Design review of the part shown in the three views and the two pictorial views. Dimensions are in mm from the part's minimum x, y and z. A direction names the side the tool comes from. Round coordinates to 2 decimals unless told otherwise and drop trailing zeros. Loops run counter-clockwise (first coordinate to the right, second up) from the corner with the lowest first, then second, coordinate; pieces in that order, holes last.
1. Consider section C-C on x = 8.25. State the section outline as (y, z) points.
2. Consider section B-B on x = 18. State the section outline as (y, z) points.
3. Clearance check with flat-ended pins moving along their axes: pin 1 Ø2.5 at (y, z) = (13, 5) entering from -X; pin 2 Ø2.5 at (x, z) = (19, 3) entering from +Y. State where each tip first meets the part, or that it passes through.
4. Consider section A-A on z = 5. State the section outline as (x, y) points, then the cut area to 3 significant figures.
5. Draft analysis for pull direction Z (two halves, no side actions). For the marked faces 4, 5 and 6, state which applies: released by +Z, released by -Z, zero draft, split by the parting line, or undercut.
6. Tool access review of the marked faces 1, 2 and 3: name each direction out of +Z, -Z, +X, -X, +Y, -Y from which nothing blocks a thin tool from reaching the whole face with its end or side.
7. To check wall thickness, follow line 1 along X through (y, z) = (3.8, 5); line 2 along Z through (x, y) = (18, 3.4); line 3 along Y through (x, z) = (11.5, 5). State the ranges of each line that lie inside material, in increasing order.
8. Consider section D-D on y = 13. State the section outline as (x, z) points, then the cut area to 3 significant figures.
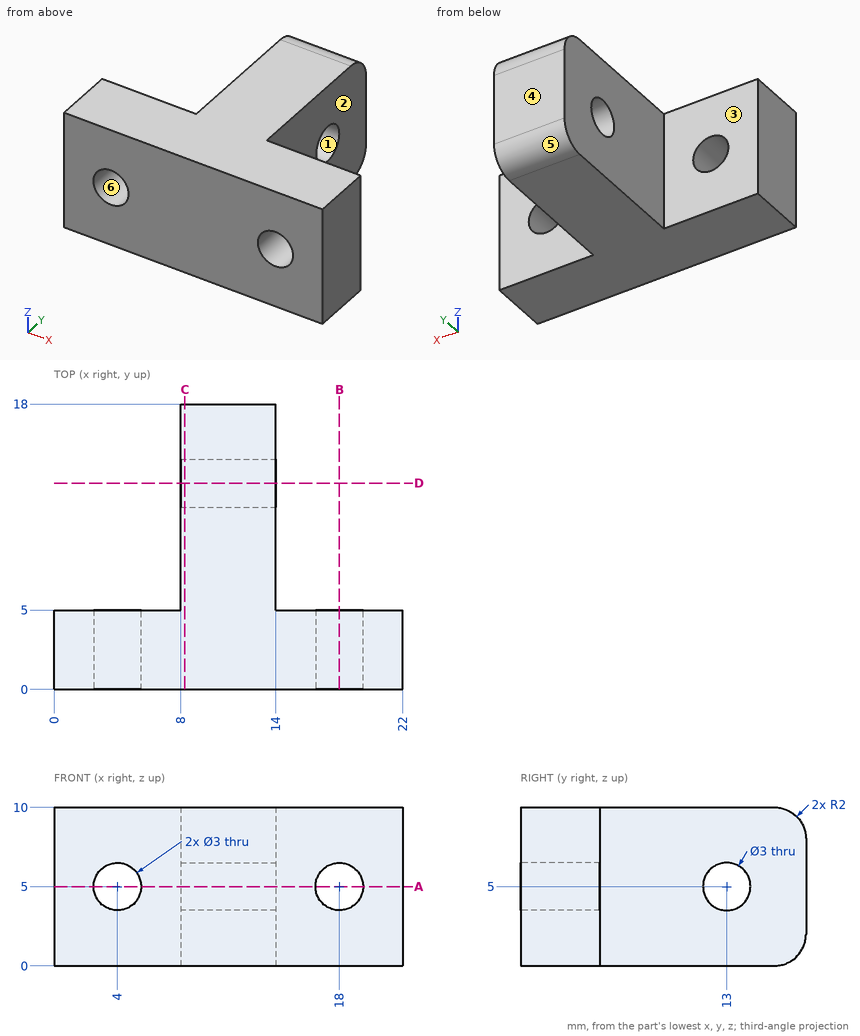
Resolved:
1. outline: (0, 0) - (16, 0) arc R2 ccw to (18, 2) - (18, 8) arc R2 ccw to (16, 10) - (0, 10) - close; hole circle Ø3 at (13, 5)
2. outline: (0, 0) - (5, 0) - (5, 3.5) - (0, 3.5) - close; (0, 6.5) - (5, 6.5) - (5, 10) - (0, 10) - close
3. pin 1: passes through
3. pin 2: stops at y = 5
4. outline: (0, 0) - (2.5, 0) - (2.5, 5) - (0, 5) - close; (5.5, 0) - (16.5, 0) - (16.5, 5) - (14, 5) - (14, 11.5) - (8, 11.5) - (8, 5) - (5.5, 5) - close; (8, 14.5) - (14, 14.5) - (14, 18) - (8, 18) - close; (19.5, 0) - (22, 0) - (22, 5) - (19.5, 5) - close
4. area: 140 mm2
5. face 4: zero draft
5. face 5: released by -Z
5. face 6: undercut
6. face 1: +X, -X
6. face 2: +Z, -Z, +X, +Y
6. face 3: +Z, -Z, -X, +Y
7. line 1: x = 0 to 2.5, 5.5 to 16.5, 19.5 to 22
7. line 2: z = 0 to 3.5, 6.5 to 10
7. line 3: y = 0 to 11.5, 14.5 to 18
8. outline: (8, 0) - (14, 0) - (14, 3.5) - (8, 3.5) - close; (8, 6.5) - (14, 6.5) - (14, 10) - (8, 10) - close
8. area: 42.0 mm2
